The listing builds one solid part. Answer for the finished solid, in the listing's coordinates (mm). Give positions to 0.01 mm unless a question says otherwise; leave off trailing zeros. Order: outer loops, then holes, each group sorted by start corner. A loop starts at its lowest first (then second) coordinate and runs counter-clockwise, first axis right, second up. Notation, with made-up numbers: M -2.5,73 L 30.5,73 A22 ccw 30.5,108 Z; hole C -28.5,42.25 d5. An arc over 180 degrees is marked long. Answer as a JSON object with one key per item and string values. Group by question number.
```python
from build123d import *

# Parameters (mm, degrees)
SKETCH1_R               = 68.25
SKETCH1_R_2             = 65.25
BOSS_EXTRUDE1_DEPTH     = 99
SKETCH2_R               = 2
CUT_EXTRUDE1_DEPTH      = 44.106233808
CUT_EXTRUDE1_DEPTH_BACK = 144.356233808
SKETCH3_R               = 2
CUT_EXTRUDE2_DEPTH      = 19.1250001
CUT_EXTRUDE2_DEPTH_BACK = 119.3750001
SKETCH4_R               = 2
CUT_EXTRUDE3_DEPTH      = 48.356233952
CUT_EXTRUDE3_DEPTH_BACK = 140.106233952


with BuildPart() as part:
    # Sketch1 → Boss-Extrude1 (new body)
    with BuildSketch(Plane.XY):
        Circle(SKETCH1_R)
        Circle(SKETCH1_R_2, mode=Mode.SUBTRACT)
    extrude(amount=-BOSS_EXTRUDE1_DEPTH)

    # Sketch2 → Cut-Extrude1 (cut, two sides)
    with BuildSketch(Plane(origin=(41.534523365, -28.310095264, -87.5), x_dir=(0, 0, -1), z_dir=(0.866025404, -0.5, 0))) as cut_extrude1_sk:
        with Locations((-4, 3.75)):
            Circle(SKETCH2_R)
        with Locations((-72, 3.75)):
            Circle(SKETCH2_R)
    extrude(amount=CUT_EXTRUDE1_DEPTH, mode=Mode.SUBTRACT)
    extrude(cut_extrude1_sk.sketch, amount=-CUT_EXTRUDE1_DEPTH_BACK, mode=Mode.SUBTRACT)

    # Sketch3 → Cut-Extrude2 (cut, two sides)
    with BuildSketch(Plane(origin=(3.75, 50.125, -87.5), x_dir=(1, 0, 0), z_dir=(0, 1, 0))) as cut_extrude2_sk:
        with Locations((-3.75, -4)):
            Circle(SKETCH3_R)
        with Locations((-3.75, -72)):
            Circle(SKETCH3_R)
    extrude(amount=CUT_EXTRUDE2_DEPTH, mode=Mode.SUBTRACT)
    extrude(cut_extrude2_sk.sketch, amount=-CUT_EXTRUDE2_DEPTH_BACK, mode=Mode.SUBTRACT)

    # Sketch4 → Cut-Extrude3 (cut, two sides)
    with BuildSketch(Plane(origin=(41.603915399, 19.689904736, -87.5), x_dir=(0, 0, -1), z_dir=(0.866025404, 0.5, 0))) as cut_extrude3_sk:
        with Locations((-4, 3.75)):
            Circle(SKETCH4_R)
        with Locations((-72, 3.75)):
            Circle(SKETCH4_R)
    extrude(amount=CUT_EXTRUDE3_DEPTH, mode=Mode.SUBTRACT)
    extrude(cut_extrude3_sk.sketch, amount=-CUT_EXTRUDE3_DEPTH_BACK, mode=Mode.SUBTRACT)


solid = part.part
```
Item 1: Determine the mould class of faces 1 (the flat face through (55.3, -35.1, -99)), 2 (the cylindrical face through (-0.26, 66.713, -85.483)), 3 (the flat face through (55.3, -35.1, 0)) for opening direction Z: released by +Z, released by -Z, zero draft, split by the parting line, or undercut.
Item 2: Consider probe 1 along Z at (x, y) = (0, -66); probe 2 along Y at (x, z) = (0, -27); probe 3 along Y at (x, z) = (29, -49.5). Determine where each line is inside the solid, lowest interval first. Write a range as from..to.
Item 3: Section C-C (x = 49.5) is taken. Determine the outline of the cut face in (y, z), and give its area (3 significant figures).
Item 4: Flat-ended cylindrical pins translate along their axes: P1, Ø6.5, axis at x = 0, z = -83.5, coming from the -Y side; P2, Ø1, axis at y = 41, z = -53.5, coming from the +X side; P3, Ø3.5, axis at x = 0, z = -15.5, coming from the -Y side; P4, Ø1, axis at x = 33.5, z = -50, coming from the +Y side. Find the tip coordinate at first contact, or state that the pin passes through.
Item 5: Section A-A (x = 0) is taken. Determine the outline of the cut face in (y, z).
Item 6: Section B-B (y = 0) is taken. Determine the outline of the cut face in (x, z), and give its area (3 significant figures).
Item 7: Section D-D (z = -15.5) is taken. Determine the outline of the cut face in (x, y), and give its area (3 significant figures).
Values found:
{
 "1": {"face 1": "released by -Z", "face 2": "undercut", "face 3": "released by +Z"},
 "2": {"probe 1": "z = -99..-85.5, -81.5..-17.5, -13.5..0", "probe 2": "y = -68.25..-65.25, 65.25..68.25", "probe 3": "y = -61.78..-58.45, 58.45..61.78"},
 "3": {"outline": "M -46.99,-99 L -42.51,-99 L -42.51,0 L -46.99,0 Z; M 42.51,-99 L 46.99,-99 L 46.99,0 L 42.51,0 Z", "area": "886 mm^2"},
 "4": {"P1": "stops at y = -68.25", "P2": "stops at x = 54.93", "P3": "passes through", "P4": "stops at y = 59.74"},
 "5": {"outline": "M -68.25,-99 L -65.25,-99 L -65.25,-85.5 L -68.25,-85.5 Z; M -68.25,-81.5 L -65.25,-81.5 L -65.25,-17.5 L -68.25,-17.5 Z; M -68.25,-13.5 L -65.25,-13.5 L -65.25,0 L -68.25,0 Z; M 65.25,-99 L 68.25,-99 L 68.25,-85.5 L 65.25,-85.5 Z; M 65.25,-81.5 L 68.25,-81.5 L 68.25,-17.5 L 65.25,-17.5 Z; M 65.25,-13.5 L 68.25,-13.5 L 68.25,0 L 65.25,0 Z"},
 "6": {"outline": "M -68.25,-99 L -65.25,-99 L -65.25,0 L -68.25,0 Z; M 65.25,-99 L 68.25,-99 L 68.25,0 L 65.25,0 Z", "area": "594 mm^2"},
 "7": {"outline": "M -60.08,-32.38 L -57.48,-30.88 A65.25 cw -57.48,30.88 L -60.08,32.38 A68.25 ccw Z; M -58.08,-35.84 A68.25 ccw -2,-68.22 L -2,-65.22 A65.25 cw -55.48,-34.34 Z; M -58.08,35.84 L -55.48,34.34 A65.25 cw -2,65.22 L -2,68.22 A68.25 ccw Z; M 2,-68.22 A68.25 ccw 58.08,-35.84 L 55.48,-34.34 A65.25 cw 2,-65.22 Z; M 2,65.22 A65.25 cw 55.48,34.34 L 58.08,35.84 A68.25 ccw 2,68.22 Z; M 57.48,-30.88 L 60.08,-32.38 A68.25 ccw 60.08,32.38 L 57.48,30.88 A65.25 cw Z", "area": "1,190 mm^2"}
}
